Verification items for the finished model (mm, model axes). Face numbers are marked on the shaded views. A direction names the side the tool comes from. Round coordinates to 2 decimals unless told otherwise and drop trailing zeros. Order: outer loops, then holes, each group sorted by start corner. A loop starts at its lowest first (then second) coordinate and runs counter-clockwise, first axis right, second up. Notation, with made-up numbers: M 88,89 L 141,89 A31 ccw 141,127 Z; hole C 6.25,-1.5 d7. An arc over 180 degrees is marked long. Use CSV: the item, a comma, the result in double quotes. Start each with the question number.
Q1. Sectioned sample at C-C (x = 4.75). Enter the section's corners in (y, z).
Q2. Sectioned sample at D-D (z = -7.75). Enter the section's corners in (x, y), and give its area (3 significant figures).
Q3. Sectioned sample at B-B (x = 13.25). Enter the section's corners in (y, z).
Q4. Sectioned sample at A-A (z = -6). Enter the section's corners in (x, y), and give its area (3 significant figures).
Q5. Set-up check for the marked faces 1, 2 and 3: record each of +Z, -Z, +X, -X, +Y, -Y from which the full face is reachable in a straight line by a thin tool's end or side.
Q6. Scan lines: line 1 (Y direction, x = 6.5, z = -7); line 2 (Y direction, x = 18.25, z = -6); line 3 (X direction, y = 23.5, z = -4.5). Record each from-to range of solid material in increasing order.
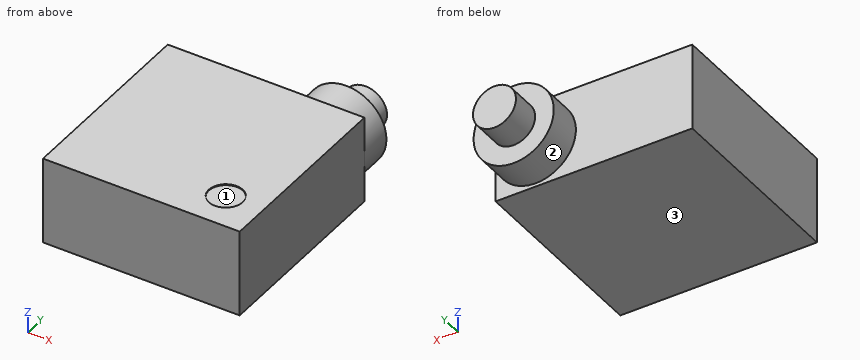
```python
from build123d import *

# Parameters (mm, degrees)
SKETCH1_W           = 19.9
SKETCH1_H           = 8.8
BOSS_EXTRUDE1_DEPTH = 19.8
SKETCH2_R           = 2.172092228
BOSS_EXTRUDE2_DEPTH = 6.55
SKETCH3_R           = 4.06071901
BOSS_EXTRUDE3_DEPTH = 3.5
SKETCH4_R           = 1.716021907
CUT_EXTRUDE1_DEPTH  = 0.1


with BuildPart() as part:
    # Sketch1 → Boss-Extrude1 (new body)
    with BuildSketch(Plane(origin=(0, 0, 0), x_dir=(1, 0, 0), z_dir=(0, 1, 0))):
        with Locations((9.95, 4.4)):
            Rectangle(SKETCH1_W, SKETCH1_H)
    extrude(amount=BOSS_EXTRUDE1_DEPTH)

    # Sketch2 → Boss-Extrude2 (add)
    with BuildSketch(Plane(origin=(0, 19.8, 0), x_dir=(1, 0, 0), z_dir=(0, 1, 0))):
        with Locations((15.83928099, 4.4)):
            Circle(SKETCH2_R)
    extrude(amount=BOSS_EXTRUDE2_DEPTH)

    # Sketch3 → Boss-Extrude3 (add)
    with BuildSketch(Plane(origin=(0, 19.8, 0), x_dir=(1, 0, 0), z_dir=(0, 1, 0))):
        with Locations((15.83928099, 4.4)):
            Circle(SKETCH3_R)
    extrude(amount=BOSS_EXTRUDE3_DEPTH)

    # Sketch4 → Cut-Extrude1 (cut)
    with BuildSketch(Plane.XY):
        with Locations((16.089426616, 3.774002994)):
            Circle(SKETCH4_R)
    extrude(amount=-CUT_EXTRUDE1_DEPTH, mode=Mode.SUBTRACT)


solid = part.part
```
Verdict:
1,outline,"M 0,-8.8 L 19.8,-8.8 L 19.8,0 L 0,0 Z"
2,outline,"M 0,0 L 19.9,0 L 19.9,19.8 L 18.13,19.8 L 18.13,23.3 L 13.54,23.3 L 13.54,19.8 L 0,19.8 Z"
2,area,"410 mm²"
3,outline,"M 0,-8.8 L 19.8,-8.8 L 19.8,-7.53 L 23.3,-7.53 L 23.3,-1.27 L 19.8,-1.27 L 19.8,0 L 0,0 Z"
4,outline,"M 0,0 L 19.9,0 L 19.9,19.8 L 19.57,19.8 L 19.57,23.3 L 17.31,23.3 L 17.31,26.35 L 14.37,26.35 L 14.37,23.3 L 12.11,23.3 L 12.11,19.8 L 0,19.8 Z"
4,area,"429 mm²"
5,face 1,"+Z"
5,face 2,"+Y"
5,face 3,"-Z, +X, -X, +Y, -Y"
6,line 1,"y = 0 to 19.8"
6,line 2,"y = 0 to 23.3"
6,line 3,"x = 13.67 to 18.01"
